```python
from build123d import *

# Parameters (mm, degrees)
SKETCH_1_W           = 15
SKETCH_1_H           = 12
EXTRUDE_1_DEPTH      = 11
SHELL_1_T            = -2
SKETCH_2_W           = 12
SKETCH_2_H           = 12
EXTRUDE_2_DEPTH      = 8
SKETCH_3_W           = 7
SKETCH_3_H           = 10
CUT_EXTRUDE_1_DEPTH  = 8
FILLET_1_R           = 0.5
SKETCH_4_W           = 5
SKETCH_4_H           = 12
EXTRUDE_3_DEPTH      = 5
EXTRUDE_4_DEPTH      = 6
EXTRUDE_4_DEPTH_BACK = 6
FILLET_2_R           = 1
FILLET_3_R           = 1
FILLET_4_R           = 0.5


with BuildPart() as part:
    # 草图1 → 凸台-拉伸1 (new body)
    with BuildSketch(Plane.XY):
        Rectangle(SKETCH_1_W, SKETCH_1_H)
    extrude(amount=EXTRUDE_1_DEPTH)

    # 抽壳1
    shell_1_openings = [part.faces().sort_by_distance(p)[0] for p in [
        (0, 0, 0),
    ]]
    offset(amount=SHELL_1_T, openings=shell_1_openings, kind=Kind.INTERSECTION)

    # 草图2 → 凸台-拉伸2 (add)
    with BuildSketch(Plane.XY.offset(11)):
        with Locations((-13.5, 0)):
            Rectangle(SKETCH_2_W, SKETCH_2_H)
    extrude(amount=-EXTRUDE_2_DEPTH)

    # 草图3 → 切除-拉伸1 (cut)
    with BuildSketch(Plane.ZY.offset(19.5)):
        with Locations((7.5, 0)):
            Rectangle(SKETCH_3_W, SKETCH_3_H)
    extrude(amount=-CUT_EXTRUDE_1_DEPTH, mode=Mode.SUBTRACT)

    # 圆角1
    fillet_1_edges = [part.edges().sort_by_distance(p)[0] for p in [
        (5.5, 0, 0),
        (0, 4, 0),
        (-5.5, 0, 0),
        (0, -4, 0),
        (0, -6, 0),
        (-7.5, 0, 0),
        (0, 6, 0),
        (7.5, 0, 0),
    ]]
    fillet(fillet_1_edges, radius=FILLET_1_R)

    # 草图4 → 凸台-拉伸3 (add)
    with BuildSketch(Plane.XY.offset(11)):
        with Locations((10, 0)):
            Rectangle(SKETCH_4_W, SKETCH_4_H)
    extrude(amount=-EXTRUDE_3_DEPTH)

    # 草图5 → 凸台-拉伸4 (add, two sides: drawn at the far end of the back side and taken through both)
    with BuildSketch(Plane(origin=(0, 0, 0), x_dir=(1, 0, 0), z_dir=(0, 1, 0)).offset(-EXTRUDE_4_DEPTH_BACK)):
        Polygon((21.541232037, -12.5), (27.5, -7.5), (27.5, -6), (20.041232037, -6), (12.5, -6), (12.5, -11), (20.041232037, -11), align=None)
    extrude(amount=EXTRUDE_4_DEPTH + EXTRUDE_4_DEPTH_BACK)

    # 圆角2
    fillet_2_edges = [part.edges().sort_by_distance(p)[0] for p in [
        (7.5, 0, 6),
    ]]
    fillet(fillet_2_edges, radius=FILLET_2_R)

    # 圆角3
    fillet_3_edges = [part.edges().sort_by_distance(p)[0] for p in [
        (-7.5, 0, 3),
    ]]
    fillet(fillet_3_edges, radius=FILLET_3_R)

    # 圆角4
    fillet_4_edges = [part.edges().sort_by_distance(p)[0] for p in [
        (21.541232037, 0, 12.5),
    ]]
    fillet(fillet_4_edges, radius=FILLET_4_R)


solid = part.part
```
Input: part model. Units: mm. Frame: model coordinates. A direction names the side the tool comes from. Give positions to 0.01 mm unless a question says otherwise; leave off trailing zeros. Order: outer loops, then holes, each group sorted by start corner. A loop starts at its lowest first (then second) coordinate and runs counter-clockwise, first axis right, second up. Notation, with made-up numbers: M 19,40.5 L 52,40.5 A25 ccw 52,53.5 Z; hole C 6,3 d6. An arc over 180 degrees is marked long. One line per question, with ' | ' between items. Start each with the question number.
1. Section query A-A (z = 1.25). Return the cut outline in (x, y).
2. Section query C-C (y = -2.5). Return the cut outline in (x, z), and give its area (3 significant figures).
3. Section query B-B (x = -2). Return the cut outline in (y, z).
4. Access query for faces 1 (the face through (0, -4, 5)), 2 (the face through (-16, 5, 7)), 3 (the face through (7.5, 0, 3)), 4 (the face through (4, 0, 11)), 5 (the face through (-14, 0, 3)). Directions: +Z, -Z, +X, -X, +Y, -Y. A direction counts if a zero-diameter tool reaches every point of the face in a straight line with its end or side. Return the directions, or none.
5. First-contact query: pin 1 Ø6.5 at (x, y) = (1.5, 1) entering from -Z; pin 2 Ø2 at (y, z) = (-2, 2.5) entering from +X; pin 3 Ø3.5 at (x, y) = (14.5, -1.5) entering from -Z. Flat tips, straight axial feed; report the tip coordinate or a pass-through.
6. Section query D-D (z = 6.75). Return the cut outline in (x, y), and give its area (3 significant figures).
7. Material intervals for probe 1 along Y at (x, z) = (0.5, 5); probe 2 along X at (y, z) = (1.5, 2); probe 3 along X at (y, z) = (-2.5, 4.5), sorted ascending. Write a range as [from, to].
Here are the results:
1) outline: M -7.5,-6 L 7.5,-6 L 7.5,6 L -7.5,6 Z; hole M -5.5,-4 L 5.5,-4 L 5.5,4 L -5.5,4 Z
2) outline: M -19.5,3 L -8.5,3 A1 cw -7.5,2 L -7.5,0.5 A0.5 ccw -7,0 L -6,0 A0.5 ccw -5.5,0.5 L -5.5,9 L 5.5,9 L 5.5,0.5 A0.5 ccw 6,0 L 7,0 A0.5 ccw 7.5,0.5 L 7.5,5 A1 cw 8.5,6 L 27.5,6 L 27.5,7.5 L 21.89,12.21 A0.5 ccw 21.22,12.18 L 20.04,11 L -11.5,11 L -11.5,4 L -19.5,4 Z | area: 201 mm²
3) outline: M -6,0.5 A0.5 ccw -5.5,0 L -4.5,0 A0.5 ccw -4,0.5 L -4,9 L 4,9 L 4,0.5 A0.5 ccw 4.5,0 L 5.5,0 A0.5 ccw 6,0.5 L 6,11 L -6,11 Z
4) face 1: -Z | face 2: +Z, -X | face 3: -Z, +X, +Y, -Y | face 4: +Z, -X, +Y, -Y | face 5: -Z, -X, +Y, -Y
5) pin 1: z = 0.07 | pin 2: x = 7.5 | pin 3: z = 6
6) outline: M -19.5,-6 L 27.5,-6 L 27.5,6 L -19.5,6 L -19.5,5 L -11.5,5 L -11.5,-5 L -19.5,-5 Z; hole M -5.5,-4 L 5.5,-4 L 5.5,4 L -5.5,4 Z | area: 396 mm²
7) probe 1: [-6, -4], [4, 6] | probe 2: [-7.5, -5.5], [5.5, 7.5] | probe 3: [-11.5, -5.5], [5.5, 7.5]
